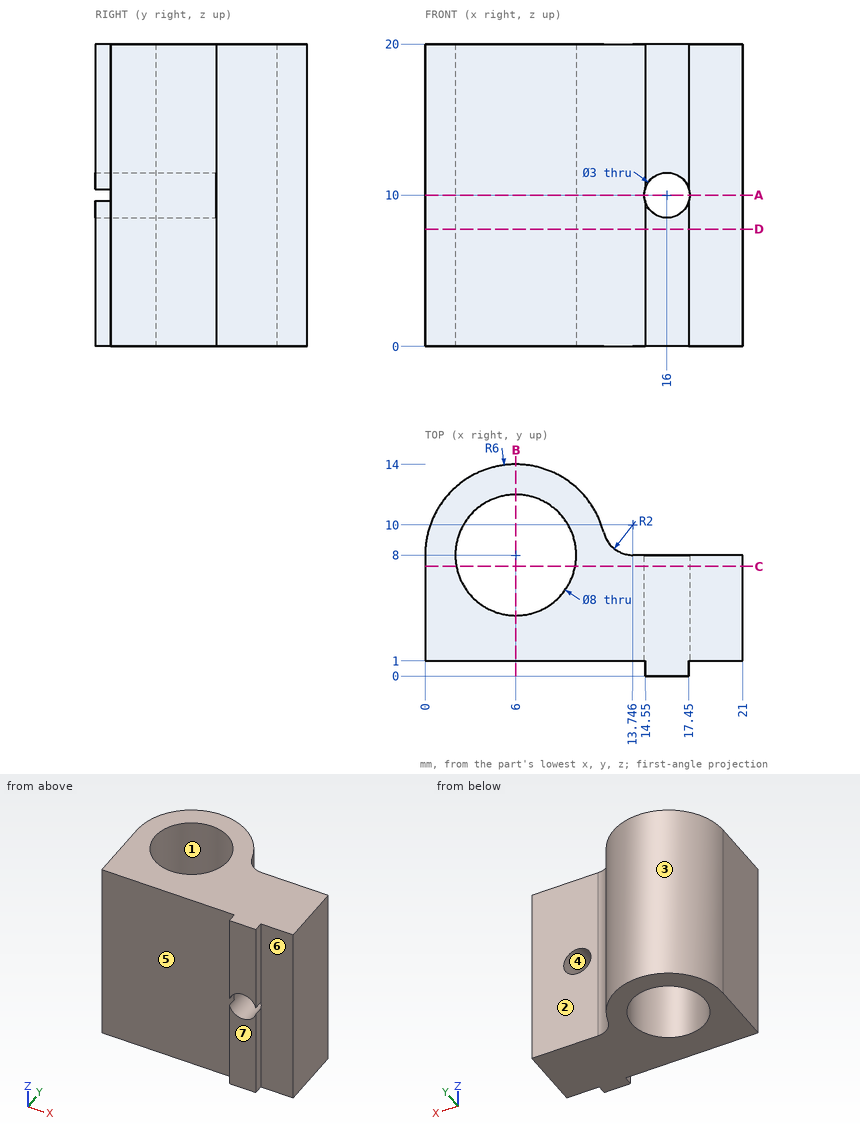
Can you work these out from the drawing? Everything is in mm from the part's minimum corner. A direction names the side the tool comes from. Give positions to 0.01 mm unless a question says otherwise; leave off trailing zeros. Write each loop counter-clockwise with the first axis right and the second up, starting at its lowest first coordinate (ties: lowest second). Pieces come first, ordered by that corner, then holes. Notation, with made-up numbers: M -36,8 L -20,8 A25 ccw -20,30 Z; hole C 3,-10 d6. An arc over 180 degrees is marked long. Answer in a Markdown table with one row per item. Add a question column.
Item 1: Imagine slicing it at A-A, the plane z = 10. Write out the boundary of the cut face in (x, y).
Item 2: Imagine slicing it at B-B, the plane x = 6. Write out the boundary of the cut face in (y, z).
Item 3: For pin 1 Ø4 at (x, z) = (5, 14.5) entering from -Y; pin 2 Ø2 at (x, z) = (3, 12) entering from +Y; pin 3 Ø6 at (x, z) = (16, 13) entering from +Y, each with a flat end and sliding along its axis, tell me the tip position at first contact or that it passes through.
Item 4: Imagine slicing it at D-D, the plane z = 7.75. Write out the boundary of the cut face in (x, y), plus the area to 3 significant figures.
Item 5: We'd pull the mould along X, two halves only. Please class the marked faces 1, 2, 3 and 4: released by +X, released by -X, zero draft, split by the parting line, or undercut.
Item 6: Imagine slicing it at C-C, the plane y = 7.25. Write out the boundary of the cut face in (x, z), plus the area to 3 significant figures.
Item 7: Please list where these lines run through material, in increasing order: L1, parallel to X at y = 3.5, z = 10; L2, parallel to Y at x = 6, z = 8.5; L3, parallel to Z at x = 16, y = 2.75.
Item 8: On a 3-axis mill with a long thin cutter (end or side, diameter ignored), from which of +Z, -Z, +X, -X, +Y, -Y can I reach the whole of each face in a straight line? I mean the marked faces 5, 6 and 7. Say none if no direction works.
Evaluation:
| question | item | result |
|---|---|---|
| 1 | outline | M 0,1 L 14.5,1 L 14.5,8 L 13.75,8 A2 cw 11.81,9.5 A6 ccw 0,8 Z; M 17.5,1 L 21,1 L 21,8 L 17.5,8 Z; hole C 6,8 d8 |
| 2 | outline | M 1,0 L 4,0 L 4,20 L 1,20 Z; M 12,0 L 14,0 L 14,20 L 12,20 Z |
| 3 | pin 1 | stops at y = 1 |
| 3 | pin 2 | stops at y = 13.66 |
| 3 | pin 3 | stops at y = 8.14 |
| 4 | outline | M 0,1 L 14.55,1 L 14.55,0 L 17.45,0 L 17.45,1 L 21,1 L 21,8 L 13.75,8 A2 cw 11.81,9.5 A6 ccw 0,8 Z; hole C 6,8 d8 |
| 4 | area | 157 mm² |
| 5 | face 1 | undercut |
| 5 | face 2 | zero draft |
| 5 | face 3 | split by the parting line |
| 5 | face 4 | undercut |
| 6 | outline | M 0,0 L 2.07,0 L 2.07,20 L 0,20 Z; M 9.93,0 L 21,0 L 21,20 L 9.93,20 Z; hole C 16,10 d3 |
| 6 | area | 256 mm² |
| 7 | L1 | x = 0 to 14.5, 17.5 to 21 |
| 7 | L2 | y = 1 to 4, 12 to 14 |
| 7 | L3 | z = 0 to 8.5, 11.5 to 20 |
| 8 | face 5 | +Z, -Z, -X, -Y |
| 8 | face 6 | +Z, -Z, +X, -Y |
| 8 | face 7 | +Z, -Z, +X, -X, -Y |
